```python
from build123d import *

# Parameters (mm, degrees)
BOSS_EXTRUDE1_DEPTH = 3
SKETCH2_R           = 5
CUT_EXTRUDE1_DEPTH  = 3
SKETCH4_R           = 5
BOSS_EXTRUDE2_DEPTH = 3
BOSS_EXTRUDE3_START = -3
SKETCH5_R           = 5
BOSS_EXTRUDE3_DEPTH = 3


with BuildPart() as part:
    # Sketch1 → Boss-Extrude1 (new body)
    with BuildSketch(Plane(origin=(0, 0, 0), x_dir=(1, 0, 0), z_dir=(0, 1, 0))):
        Polygon((0, 0), (40.989942652, -0.908075633), (41.875870099, 39.082112321), (0.885927446, 39.990187954), align=None)
    extrude(amount=BOSS_EXTRUDE1_DEPTH)

    # Sketch2 → Cut-Extrude1 (cut)
    with BuildSketch(Plane(origin=(0, 3, 0), x_dir=(1, 0, 0), z_dir=(0, 1, 0))):
        with Locations(Location((20.937935049, 19.54105616, 0), (0, 0, 270))):
            Circle(SKETCH2_R)
    extrude(amount=-CUT_EXTRUDE1_DEPTH, mode=Mode.SUBTRACT)

    # Sketch4 → Boss-Extrude2 (add)
    with BuildSketch(Plane(origin=(0, 0, 0), x_dir=(0.9997546988385365, 0, 0.022148186162014694), z_dir=(-0.02214818616201469, 0, 0.9997546988385364))):
        with BuildLine():
            Line((41, 15.324050928), (41, 3))
            Line((41, 3), (0, 3))
            Line((0, 3), (0, 15.324050928))
            ThreePointArc((0, 15.324050928), (20.5, 35.824050928), (41, 15.324050928))
        make_face()
        with Locations((20.5, 15.324050928)):
            Circle(SKETCH4_R, mode=Mode.SUBTRACT)
    extrude(amount=-BOSS_EXTRUDE2_DEPTH)

    # Sketch5 → Boss-Extrude3 (add)
    with BuildSketch(Plane(origin=(0.885927446, 0, -39.990187954), x_dir=(-0.9997546988385365, 0, -0.022148186162014458), z_dir=(0.022148186162014454, 0, -0.9997546988385364)).offset(BOSS_EXTRUDE3_START)):
        with BuildLine():
            Line((-41, 3), (-41, 15.324050928))
            ThreePointArc((-41, 15.324050928), (-20.5, 35.824050928), (0, 15.324050928))
            Line((0, 15.324050928), (0, 3))
            Line((0, 3), (-41, 3))
        make_face()
        with Locations(Location((-20.5, 15.324050928, 0), (0, 0, 180))):
            Circle(SKETCH5_R, mode=Mode.SUBTRACT)
    extrude(amount=BOSS_EXTRUDE3_DEPTH)


solid = part.part
```
The listing builds one solid part. Answer for the finished solid, in the listing's coordinates (mm). A direction names the side the tool comes from. Coordinates: 2 decimals unless noted, no trailing zeros. Order: outer loops, then holes, each group sorted by start corner. A loop starts at its lowest first (then second) coordinate and runs counter-clockwise, first axis right, second up. Notation, with made-up numbers: M 54.25,54 L 71.25,54 A24 cw 71.25,77 Z; hole C 74,-33 d9. An arc over 180 degrees is marked long. Answer as a JSON object with one key per item and string values. Group by question number.
1. Straight lines are drawn through the part: line 1 (Y direction, x = 23, z = -35); line 2 (Z direction, x = 8, y = 11); line 3 (Z direction, x = 26, y = 21.5). For each, find the intervals that lie inside material, in ascending order.
2. Section C-C on z = -19.5 is taken. Write down the section's boundary in (x, y).
3. Flat-ended cylindrical pins translate along their axes: P1, Ø5, axis at x = 31, y = 4.5, coming from the -Z side; P2, Ø2, axis at x = 6, z = -30.5, coming from the +Y side; P3, Ø3, axis at x = 22, y = 17, coming from the -Z side; P4, Ø2, axis at x = 31.5, y = 15, coming from the -Z side. Find the tip coordinate at first contact, or state that the pin passes through.
4. A tool of negligible diameter and unlimited length cuts with its end or side. For faces 1 (the cylindrical face through (22.44, 1.52, -14.77)), 2 (the cylindrical face through (20.08, 35.82, -1.03)), 3 (the cylindrical face through (19.88, 20.28, -1.04)), from which of +Z, -Z, +X, -X, +Y, -Y can it reach the whole face along a straight path? Write none if from no direction.
5. Section A-A on y = 28.5 is taken. Write down the section's boundary in (x, z), then the cut area to 3 significant figures.
6. Section D-D on x = 21.5 is taken. State how many separate pieces and enclosed holes the cut face has, then the cut area to 3 significant figures.
7. Determine the mould class of faces 4 (the cylindrical face through (21.8, 35.82, -38.01)), 5 (the flat face through (25, 0, -24)), 6 (the cylindrical face through (20.264, 20.205, -38.04)) for opening direction Y: released by +Y, released by -Y, zero draft, split by the parting line, or undercut.
8. Section B-B on y = 18 is taken. Write down the section's boundary in (x, z).
Values follow:
{
 "1": {"line 1": "0 to 3", "line 2": "-39.83 to -36.83, -2.82 to 0.18", "line 3": "-39.43 to -36.43, -2.42 to 0.58"},
 "2": {"outline": "M 0.43,0 L 15.94,0 L 15.94,3 L 0.43,3 Z; M 25.94,0 L 41.44,0 L 41.44,3 L 25.94,3 Z"},
 "3": {"P1": "z = -39.38", "P2": "y = 3", "P3": "through", "P4": "z = -39.33"},
 "4": {"face 1": "+Y, -Y", "face 2": "+Y", "face 3": "none"},
 "5": {"outline": "M 4.79,0.11 L 4.86,-2.89 L 36.26,-2.2 L 36.2,0.8 Z; M 5.61,-36.88 L 5.68,-39.88 L 37.08,-39.19 L 37.02,-36.19 Z", "area": "188 mm2"},
 "6": {"separate pieces": "4", "enclosed holes": "0", "area": "228 mm2"},
 "7": {"face 4": "released by +Y", "face 5": "released by -Y", "face 6": "undercut"},
 "8": {"outline": "M 0.18,0 L 0.24,-3 L 16.34,-2.64 L 16.27,0.36 Z; M 0.99,-36.99 L 1.06,-39.99 L 17.16,-39.63 L 17.09,-36.63 Z; M 24.72,0.55 L 24.78,-2.45 L 40.88,-2.1 L 40.81,0.9 Z; M 25.54,-36.44 L 25.6,-39.44 L 41.7,-39.09 L 41.63,-36.09 Z"}
}
